Verification items for the finished model (mm, model axes). Face numbers are marked on the shaded views. A direction names the side the tool comes from. Give positions to 0.01 mm unless a question says otherwise; leave off trailing zeros. Write each loop counter-clockwise with the first axis right and the second up, starting at its lowest first coordinate (ties: lowest second). Pieces come first, ordered by that corner, then holes. Notation, with made-up numbers: (-1.75, 86) - (46.25, 86) arc R32 ccw to (46.25, 113) - close; hole circle Ø7 at (34.25, 51). An arc over 180 degrees is marked (long way). Put each result on its own line as item: value.
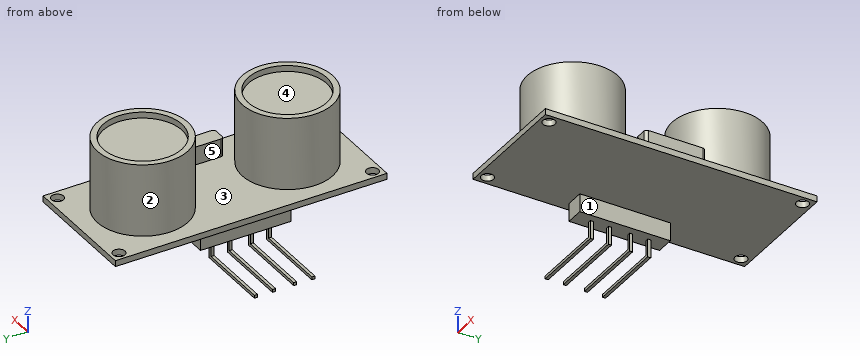
from build123d import *

# Parameters (mm, degrees)
SKETCH1_W           = 20
SKETCH1_H           = 45
BOSS_EXTRUDE1_DEPTH = 1
SKETCH2_R           = 7.5
BOSS_EXTRUDE2_DEPTH = 12
SKETCH3_R           = 6.5
CUT_EXTRUDE1_DEPTH  = 1
SKETCH4_W           = 2.6
SKETCH4_H           = 10
BOSS_EXTRUDE3_DEPTH = 3
FILLET1_R           = 0.5
SKETCH5_W           = 3
SKETCH5_H           = 15
BOSS_EXTRUDE4_DEPTH = 3
SKETCH6_W           = 0.5
SKETCH6_H           = 0.5
BOSS_EXTRUDE5_DEPTH = 3
SKETCH7_W           = 0.490041207
SKETCH7_H           = 0.5
BOSS_EXTRUDE6_DEPTH = 12
SKETCH8_R           = 1
CUT_EXTRUDE2_DEPTH  = 3


with BuildPart() as part:
    # Sketch1 → Boss-Extrude1 (new body)
    with BuildSketch(Plane.XY):
        with Locations((-12.292244857, -79.882705913)):
            Rectangle(SKETCH1_W, SKETCH1_H)
    extrude(amount=BOSS_EXTRUDE1_DEPTH)

    # Sketch2 → Boss-Extrude2 (add)
    with BuildSketch(Plane.XY.offset(1)):
        with Locations((-12.292244857, -67.882705913)):
            Circle(SKETCH2_R)
        with Locations((-12.292244857, -91.882705913)):
            Circle(SKETCH2_R)
    extrude(amount=BOSS_EXTRUDE2_DEPTH)

    # Sketch3 → Cut-Extrude1 (cut)
    with BuildSketch(Plane.XY.offset(13)):
        with Locations((-12.292244857, -67.882705913)):
            Circle(SKETCH3_R)
        with Locations((-12.292244857, -91.882705913)):
            Circle(SKETCH3_R)
    extrude(amount=-CUT_EXTRUDE1_DEPTH, mode=Mode.SUBTRACT)

    # Sketch4 → Boss-Extrude3 (add)
    with BuildSketch(Plane.XY.offset(1)):
        with Locations((-5.092244857, -79.882705913)):
            Rectangle(SKETCH4_W, SKETCH4_H)
    extrude(amount=BOSS_EXTRUDE3_DEPTH)

    # Fillet1
    fillet1_edges = [part.edges().sort_by_distance(p)[0] for p in [
        (-6.392244857, -74.882705913, 2.5),
        (-6.392244857, -84.882705913, 2.5),
        (-3.792244857, -84.882705913, 2.5),
        (-3.792244857, -74.882705913, 2.5),
    ]]
    fillet(fillet1_edges, radius=FILLET1_R)

    # Sketch5 → Boss-Extrude4 (add)
    with BuildSketch(Plane(origin=(0, 0, 0), x_dir=(-1, 0, 0), z_dir=(0, 0, -1))):
        with Locations((19.292244857, -79.882705913)):
            Rectangle(SKETCH5_W, SKETCH5_H)
    extrude(amount=BOSS_EXTRUDE4_DEPTH)

    # Sketch6 → Boss-Extrude5 (add)
    with BuildSketch(Plane(origin=(0, 0, -3), x_dir=(-1, 0, 0), z_dir=(0, 0, -1))):
        with Locations((19.292244857, -84.632705913)):
            Rectangle(SKETCH6_W, SKETCH6_H)
        with Locations((19.292244857, -81.632705913)):
            Rectangle(SKETCH6_W, SKETCH6_H)
        with Locations((19.292244857, -78.132705913)):
            Rectangle(SKETCH6_W, SKETCH6_H)
        with Locations((19.292244857, -75.132705913)):
            Rectangle(SKETCH6_W, SKETCH6_H)
    extrude(amount=BOSS_EXTRUDE5_DEPTH)

    # Sketch7 → Boss-Extrude6 (add)
    with BuildSketch(Plane.ZY.offset(19.542244857)):
        with Locations((-5.754979396, -75.132705913)):
            Rectangle(SKETCH7_W, SKETCH7_H)
        with Locations((-5.754979396, -78.132705913)):
            Rectangle(SKETCH7_W, SKETCH7_H)
        with Locations((-5.754979396, -81.632705913)):
            Rectangle(SKETCH7_W, SKETCH7_H)
        with Locations((-5.754979396, -84.632705913)):
            Rectangle(SKETCH7_W, SKETCH7_H)
    extrude(amount=BOSS_EXTRUDE6_DEPTH)

    # Sketch8 → Cut-Extrude2 (cut)
    with BuildSketch(Plane.XY.offset(1)):
        with Locations((-20.792244857, -58.882705913)):
            Circle(SKETCH8_R)
        with Locations((-3.792244857, -58.882705913)):
            Circle(SKETCH8_R)
        with Locations((-3.792244857, -100.882705913)):
            Circle(SKETCH8_R)
        with Locations((-20.792244857, -100.882705913)):
            Circle(SKETCH8_R)
    extrude(amount=-CUT_EXTRUDE2_DEPTH, mode=Mode.SUBTRACT)


solid = part.part
Q1. Section check B-B, the plane x = -26. Record the cut outline in (y, z), plus the area to 3 significant figures.
Answers follow:
outline: (-84.88, -6) - (-84.38, -6) - (-84.38, -5.51) - (-84.88, -5.51) - close; (-81.88, -6) - (-81.38, -6) - (-81.38, -5.51) - (-81.88, -5.51) - close; (-78.38, -6) - (-77.88, -6) - (-77.88, -5.51) - (-78.38, -5.51) - close; (-75.38, -6) - (-74.88, -6) - (-74.88, -5.51) - (-75.38, -5.51) - close
area: 0.980 mm2
Q2. Section check C-C, the plane y = -80. Record the cut outline in (x, z), plus the area to 3 significant figures.
Answers follow:
outline: (-22.29, 0) - (-20.79, 0) - (-20.79, -3) - (-17.79, -3) - (-17.79, 0) - (-2.29, 0) - (-2.29, 1) - (-3.79, 1) - (-3.79, 4) - (-6.39, 4) - (-6.39, 1) - (-22.29, 1) - close
area: 36.8 mm2
Q3. Release check for a two-part mould opening along Y. For the marked faces 1, 2 and 3 record: released by +Y, released by -Y, zero draft, split by the parting line, or undercut.
Answers follow:
face 1: zero draft
face 2: undercut
face 3: undercut
Q4. Section check D-D, the plane x = -20.25. Give the number of separate pieces and of enclosed holes in the cut face, plus the area to 3 significant figures.
Answers follow:
separate pieces: 7
enclosed holes: 0
area: 87.6 mm2
Q5. Section check A-A, the plane z = -3.75. Record the cut outline in (x, y), plus the area to 3 significant figures.
Answers follow:
outline: (-19.54, -84.88) - (-19.04, -84.88) - (-19.04, -84.38) - (-19.54, -84.38) - close; (-19.54, -81.88) - (-19.04, -81.88) - (-19.04, -81.38) - (-19.54, -81.38) - close; (-19.54, -78.38) - (-19.04, -78.38) - (-19.04, -77.88) - (-19.54, -77.88) - close; (-19.54, -75.38) - (-19.04, -75.38) - (-19.04, -74.88) - (-19.54, -74.88) - close
area: 1.00 mm2
Q6. Set-up check for the marked faces 4 and 5: record each of +Z, -Z, +X, -X, +Y, -Y from which the full face is reachable in a straight line by a thin tool's end or side.
Answers follow:
face 4: +Z
face 5: +Z, -X
Q7. Scan lines: line 1 along Y through (x, z) = (-8.25, 12.25); line 2 along Z through (x, y) = (-6, -75.5); line 3 along X through (y, z) = (-87.5, 12.25). Record each from-to range of solid material in increasing order.
Answers follow:
line 1: y = -98.2 to -96.97, -86.79 to -85.57, -74.2 to -72.97, -62.79 to -61.57
line 2: z = 0 to 4
line 3: x = -18.38 to -17.09, -7.49 to -6.21
Q8. Go/stop test with flat-tipped pins: pin 1 Ø5 at (x, z) = (-16.5, 4) entering from -Y; pin 2 Ø12 at (x, y) = (-8.5, -66) entering from -Z; pin 3 Ø4 at (x, z) = (-17.5, 6) entering from -Y. Record where each tip stops, or that it passes through.
Answers follow:
pin 1: stops at y = -99.19
pin 2: stops at z = 0
pin 3: stops at y = -98.66
